Geometry check sheet. Reference: the model listing, model coordinates, mm. Face numbers are marked on the shaded views. A direction names the side the tool comes from. Round coordinates to 2 decimals unless told otherwise and drop trailing zeros. Loops run counter-clockwise (first coordinate to the right, second up) from the corner with the lowest first, then second, coordinate; pieces in that order, holes last. Notation, with made-up numbers: (48.5, 89) - (90.5, 89) arc R30 ccw to (90.5, 123) - close; hole circle Ø4 at (62.5, -8.75). An arc over 180 degrees is marked (long way). Answer in a Markdown table with one row per item. Add a question column.
```python
from build123d import *

# Parameters (mm, degrees)
CROQUIS2_W                 = 18
CROQUIS2_H                 = 15
SALIENTE_EXTRUIR1_DEPTH    = 5.5
CROQUIS3_W                 = 18
CROQUIS3_H                 = 9
CORTAR_EXTRUIR1_DEPTH      = 1.5
CORTAR_EXTRUIR2_DEPTH      = 13.942179106
CROQUIS10_W                = 6
CROQUIS10_H                = 11
SALIENTE_EXTRUIR4_DEPTH    = 10
CORTAR_EXTRUIR3_DEPTH      = 21.432816742
CORTAR_EXTRUIR3_DEPTH_BACK = 21.432816742
CROQUIS7_R                 = 1.5
CORTAR_EXTRUIR4_DEPTH      = 21.432816742
CORTAR_EXTRUIR4_DEPTH_BACK = 21.432816742
CROQUIS11_R                = 1.5
REDONDEO2_R                = 1.5
REDONDEO3_R                = 1.5
CROQUIS15_R                = 1.5
CORTAR_EXTRUIR7_DEPTH      = 10


with BuildPart() as part:
    # Croquis2 → Saliente-Extruir1 (new, symmetric)
    with BuildSketch(Plane.XY):
        Rectangle(CROQUIS2_W, CROQUIS2_H)
    extrude(amount=SALIENTE_EXTRUIR1_DEPTH, both=True)

    # Croquis3 → Cortar-Extruir1 (cut, symmetric)
    with BuildSketch(Plane.XY):
        with Locations((0, -3)):
            Rectangle(CROQUIS3_W, CROQUIS3_H)
    extrude(amount=CORTAR_EXTRUIR1_DEPTH, both=True, mode=Mode.SUBTRACT)

    # Croquis4 → Cortar-Extruir2 (cut, through all)
    with BuildSketch(Plane.XY):
        with BuildLine():
            Line((0.5, -1.5), (-0.5, -1.5))
            ThreePointArc((-0.5, -1.5), (-1.207106781, -1.792893219), (-1.5, -2.5))
            Line((-1.5, -2.5), (-1.5, -3))
            Line((-1.5, -3), (-1.5, -7.5))
            Line((-1.5, -7.5), (1.5, -7.5))
            Line((1.5, -7.5), (1.5, -3))
            Line((1.5, -3), (1.5, -2.5))
            ThreePointArc((1.5, -2.5), (1.207106781, -1.792893219), (0.5, -1.5))
        make_face()
    extrude(amount=-CORTAR_EXTRUIR2_DEPTH, mode=Mode.SUBTRACT)

    # Croquis10 → Saliente-Extruir4 (add)
    with BuildSketch(Plane(origin=(0, 7.5, 0), x_dir=(1, 0, 0), z_dir=(0, 1, 0))):
        with Locations((-6, 0)):
            Rectangle(CROQUIS10_W, CROQUIS10_H)
        with Locations((6, 0)):
            Rectangle(CROQUIS10_W, CROQUIS10_H)
    extrude(amount=SALIENTE_EXTRUIR4_DEPTH)

    # Croquis7 → Cortar-Extruir3 (cut, two sides: drawn at the far end of the back side and taken through both)
    with BuildSketch(Plane(origin=(0, 0, 0), x_dir=(0, 0, -1), z_dir=(1, 0, 0)).offset(-CORTAR_EXTRUIR3_DEPTH_BACK)):
        with Locations((0, 13.5)):
            Circle(CROQUIS7_R)
    extrude(amount=CORTAR_EXTRUIR3_DEPTH + CORTAR_EXTRUIR3_DEPTH_BACK, mode=Mode.SUBTRACT)

    # Croquis11 → Cortar-Extruir4 (cut, two sides: drawn at the far end of the back side and taken through both)
    with BuildSketch(Plane.XY.offset(-CORTAR_EXTRUIR4_DEPTH_BACK)):
        with Locations((6, -3)):
            Circle(CROQUIS11_R)
        with Locations((-6, -3)):
            Circle(CROQUIS11_R)
    extrude(amount=CORTAR_EXTRUIR4_DEPTH + CORTAR_EXTRUIR4_DEPTH_BACK, mode=Mode.SUBTRACT)

    # Redondeo2
    redondeo2_edges = [part.edges().sort_by_distance(p)[0] for p in [
        (6, 17.5, -5.5),
        (6, 17.5, 5.5),
        (-6, 17.5, 5.5),
        (-6, 17.5, -5.5),
    ]]
    fillet(redondeo2_edges, radius=REDONDEO2_R)

    # Redondeo3
    redondeo3_edges = [part.edges().sort_by_distance(p)[0] for p in [
        (9, -7.5, -3.5),
        (-9, -7.5, -3.5),
        (9, -7.5, 3.5),
        (-9, -7.5, 3.5),
    ]]
    fillet(redondeo3_edges, radius=REDONDEO3_R)

    # Croquis15 → Cortar-Extruir7 (cut)
    with BuildSketch(Plane.XY.offset(5.5)):
        with Locations((0, 5)):
            Circle(CROQUIS15_R)
    extrude(amount=-CORTAR_EXTRUIR7_DEPTH, mode=Mode.SUBTRACT)


solid = part.part
```
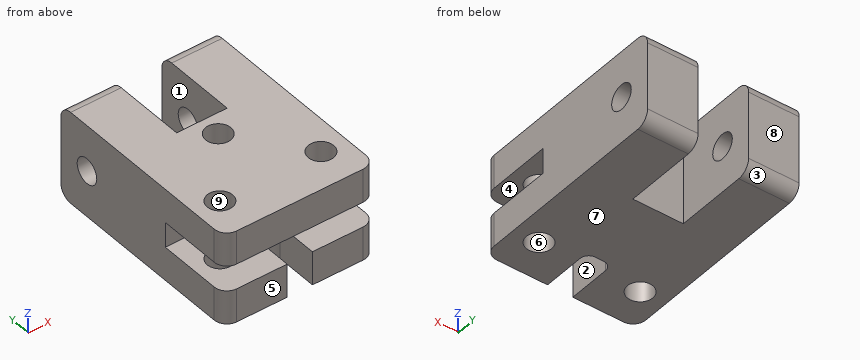
Q1. Set-up check for the marked faces 1, 2, 3, 4 and 5: record each of +Z, -Z, +X, -X, +Y, -Y from which the full face is reachable in a straight line by a thin tool's end or side.
Q2. Cross-section at A-A, the plane z = 0. Enter the section's corners in (x, y), plus the area to 3 significant figures.
Q3. Depth check by flat-ended pin: P1, Ø1.8, axis at x = 6, y = -3, coming from the -Z side; P2, Ø0.5, axis at x = 0, z = -4.5, coming from the -Y side; P3, Ø2.5, axis at x = -2.5, z = 0, coming from the -Y side; P4, Ø3, axis at x = 0, z = -1, coming from the +Y side. Enter the tip coordinate at first touch or a pass-through.
Q4. Cross-section at B-B, the plane y = 1. Enter the section's corners in (x, z), plus the area to 3 significant figures.
Q5. Scan lines: line 1 (X direction, y = -3, z = -4.25); line 2 (Y direction, x = -6, z = 3.7); line 3 (X direction, y = 11.25, z = 3.75). Record each from-to range of solid material in increasing order. Write a range as from..to.
Q6. Release check for a two-part mould opening along Y. For the marked faces 6, 7, 8 and 9 record: +Y half, -Y half, draft (parallel to the pull), parting line (faces both ways), or undercut.
Q7. Cross-section at C-C, the plane x = -6. Enter the section's corners in (y, z), plus the area to 3 significant figures.
Q8. Cross-section at D-D, the plane y = -3. Enter the section's corners in (x, z), plus the area to 3 significant figures.
Check sheet entries:
| question | item | result |
|---|---|---|
| 1 | face 1 | +Z, -Z, +Y |
| 1 | face 2 | -Z, -Y |
| 1 | face 3 | -Z, +X, -X, +Y |
| 1 | face 4 | +X, -X, -Y |
| 1 | face 5 | +Z, -Z, +X, -X, -Y |
| 2 | outline | (-9, 1.5) - (9, 1.5) - (9, 12) - (3, 12) - (3, 7.5) - (-3, 7.5) - (-3, 12) - (-9, 12) - close; (-9, 15) - (-3, 15) - (-3, 17.5) - (-9, 17.5) - close; (3, 15) - (9, 15) - (9, 17.5) - (3, 17.5) - close; hole circle Ø3 at (0, 5) |
| 2 | area | 185 mm² |
| 3 | P1 | through |
| 3 | P2 | y = -1.5 |
| 3 | P3 | y = 1.5 |
| 3 | P4 | y = 7.5 |
| 4 | outline | (-9, -5.5) - (9, -5.5) - (9, -1.5) - (-9, -1.5) - close; (-9, 1.5) - (9, 1.5) - (9, 5.5) - (-9, 5.5) - close |
| 4 | area | 144 mm² |
| 5 | line 1 | -9..-7.5, -4.5..-1.5, 1.5..4.5, 7.5..9 |
| 5 | line 2 | -7.5..-4.5, -1.5..17.5 |
| 5 | line 3 | -9..-3, 3..9 |
| 6 | face 6 | undercut |
| 6 | face 7 | draft |
| 6 | face 8 | +Y half |
| 6 | face 9 | undercut |
| 7 | outline | (-7.5, -5.5) - (-4.5, -5.5) - (-4.5, -1.5) - (-7.5, -1.5) - close; (-7.5, 1.5) - (-4.5, 1.5) - (-4.5, 5.5) - (-7.5, 5.5) - close; (-1.5, -5.5) - (16, -5.5) arc R1.5 ccw to (17.5, -4) - (17.5, 4) arc R1.5 ccw to (16, 5.5) - (-1.5, 5.5) - (-1.5, 1.5) - (1.5, 1.5) - (1.5, -1.5) - (-1.5, -1.5) - close; hole circle Ø3 at (13.5, 0) |
| 7 | area | 216 mm² |
| 8 | outline | (-9, -5.5) - (-7.5, -5.5) - (-7.5, -1.5) - (-9, -1.5) - close; (-9, 1.5) - (-7.5, 1.5) - (-7.5, 5.5) - (-9, 5.5) - close; (-4.5, -5.5) - (-1.5, -5.5) - (-1.5, -1.5) - (-4.5, -1.5) - close; (-4.5, 1.5) - (4.5, 1.5) - (4.5, 5.5) - (-4.5, 5.5) - close; (1.5, -5.5) - (4.5, -5.5) - (4.5, -1.5) - (1.5, -1.5) - close; (7.5, -5.5) - (9, -5.5) - (9, -1.5) - (7.5, -1.5) - close; (7.5, 1.5) - (9, 1.5) - (9, 5.5) - (7.5, 5.5) - close |
| 8 | area | 84.0 mm² |
